Geometry check sheet. Reference: the model listing, model coordinates, mm. A direction names the side the tool comes from. Round coordinates to 2 decimals unless told otherwise and drop trailing zeros. Loops run counter-clockwise (first coordinate to the right, second up) from the corner with the lowest first, then second, coordinate; pieces in that order, holes last.
```python
from build123d import *

# Parameters (mm, degrees)
F0_R     = 15.875
F1_DEPTH = 31.75
F2_DEPTH = 92.075
F0_W     = 31.75
F0_H     = 88.9
F3_DEPTH = 73.025
F4_DEPTH = 53.975


# Not quite as in the source:
# - a feature names something its author has since deleted; it is built from what else it names


with BuildPart() as f1:
    # F0 (on Front) → F1 (new body)
    with BuildSketch(Plane.XZ):
        Polygon((-69.8361151936, 86.826035718), (-126.218325014, 80.5985571647), (-126.4791783958, 29.7122203269), (-85.725, 29.7122203269), (-85.725, -21.0877796731), (-126.7395891979, -21.0877796731), (-127, -71.8877796731), (-69.8361151936, -65.5739758634), (-69.8361151936, -40.1377796731), (-69.8361151936, 48.7622203269), align=None)
        Polygon((126.2463778257, 108.4835678339), (-69.8361151936, 86.826035718), (-69.8361151936, 48.7622203269), (-38.0861151936, 48.7622203269), (-38.0861151936, -40.1377796731), (-38.0861151936, -62.0671590745), (38.1138848064, -53.6507987812), (38.1138848064, -40.1378311361), (38.1138848064, 48.7622203269), (69.8638848064, 48.7622203269), (69.8638848064, -40.1378311361), (69.8638848064, -50.1439819923), (126.2463778257, -43.9164836263), (126.2463778257, 6.8835678339), (85.725, 6.8835678339), (85.725, 57.6835678339), (126.2463778257, 57.6835678339), align=None)
        Circle(F0_R, mode=Mode.SUBTRACT)
        Polygon((-38.0861151936, -40.1377796731), (-69.8361151936, -40.1377796731), (-69.8361151936, -65.5739758634), (-38.0861151936, -62.0671590745), align=None)
    extrude(amount=F1_DEPTH)

    # F0 (on Front) → F2 (join)
    with BuildSketch(Plane.XZ):
        Polygon((126.2463778257, 108.4835678339), (-69.8361151936, 86.826035718), (-69.8361151936, 48.7622203269), (-38.0861151936, 48.7622203269), (-38.0861151936, -40.1377796731), (-38.0861151936, -62.0671590745), (38.1138848064, -53.6507987812), (38.1138848064, -40.1378311361), (38.1138848064, 48.7622203269), (69.8638848064, 48.7622203269), (69.8638848064, -40.1378311361), (69.8638848064, -50.1439819923), (126.2463778257, -43.9164836263), (126.2463778257, 6.8835678339), (85.725, 6.8835678339), (85.725, 57.6835678339), (126.2463778257, 57.6835678339), align=None)
        Circle(F0_R, mode=Mode.SUBTRACT)
        Polygon((-38.0861151936, -40.1377796731), (-69.8361151936, -40.1377796731), (-69.8361151936, -65.5739758634), (-38.0861151936, -62.0671590745), align=None)
        Polygon((38.1138848064, -40.1378311361), (38.1138848064, -53.6507987812), (69.8638848064, -50.1439819923), (69.8638848064, -40.1378311361), align=None)
    extrude(amount=F2_DEPTH)

    # F0 (on Front) → F3 (join)
    with BuildSketch(Plane.XZ):
        with Locations((-53.9611151936, 4.3122203269)):
            Rectangle(F0_W, F0_H)
    extrude(amount=F3_DEPTH)

    # F0 (on Front) → F4 (join)
    with BuildSketch(Plane.XZ):
        Polygon((126.2463778257, 108.4835678339), (-69.8361151936, 86.826035718), (-69.8361151936, 48.7622203269), (-38.0861151936, 48.7622203269), (-38.0861151936, -40.1377796731), (-38.0861151936, -62.0671590745), (38.1138848064, -53.6507987812), (38.1138848064, -40.1378311361), (38.1138848064, 48.7622203269), (69.8638848064, 48.7622203269), (69.8638848064, -40.1378311361), (69.8638848064, -50.1439819923), (126.2463778257, -43.9164836263), (126.2463778257, 6.8835678339), (85.725, 6.8835678339), (85.725, 57.6835678339), (126.2463778257, 57.6835678339), align=None)
        Circle(F0_R, mode=Mode.SUBTRACT)
    extrude(amount=F4_DEPTH)


solid = f1.part
```
1) Gauge pin test, flat ends, axial feed: pin 1 (21 mm diameter, centred on x = -49.5, y = -78, fed in from -Z); pin 2 (5 mm diameter, centred on x = 47.5, y = -26.5, fed in from -Z); pin 3 (16 mm diameter, centred on x = -110.5, y = -9.5, fed in from -Z). Record the tip position at first contact, or that the pin passes through.
Report:
pin 1: stops at z = -64.49
pin 2: stops at z = -52.89
pin 3: stops at z = -70.95
2) Scan lines: line 1 along X through (y, z) = (-38.5, -29); line 2 along X through (y, z) = (-46.5, -5); line 3 along X through (y, z) = (-38, -7.5). Record each from-to range of solid material in increasing order.
Report:
line 1: x = -69.84 to 38.11, 69.86 to 126.25
line 2: x = -69.84 to -15.07, 15.07 to 38.11, 69.86 to 126.25
line 3: x = -69.84 to -13.99, 13.99 to 38.11, 69.86 to 126.25
3) Mould release check, pull along Z, two halves, no side actions. Record for faces 6 (the face through (126.246, -45, -19)), 7 (the face through (-38.086, -82, 5)), 8 (the face through (25.99, -45.39, -54.99)), 9 (the face through (-85.725, -16, 5)): +Z half, -Z half, draft (parallel to the pull), parting line (faces both ways), or undercut.
Report:
face 6: draft
face 7: undercut
face 8: -Z half
face 9: undercut
4) Access from +Z, -Z, +X, -X, +Y, -Y to the whole of each face (thin tool, end or side, straight path). Record for faces 1 (the face through (-69.836, -55, 10)), 2 (the face through (54, -45, -40.138)), 3 (the face through (-54, -82, 48.762)), 4 (the face through (106, -45, 57.684)), 5 (the face through (-106, -16, -21.088)).
Report:
face 1: +Z, -Z, -X, -Y
face 2: +Y, -Y
face 3: -X, -Y
face 4: +X, +Y, -Y
face 5: -X, +Y, -Y
5) Sectioned sample at A-A, the plane y = -57.5. Record the cut outline in (x, z) (3 decimals).
Report:
outline: (-69.836, -65.574) - (126.246, -43.916) - (126.246, 6.884) - (85.725, 6.884) - (85.725, 57.684) - (126.246, 57.684) - (126.246, 108.484) - (-69.836, 86.826) - close; hole circle Ø31.75 at (0, 0); hole (38.114, -40.138) - (69.864, -40.138) - (69.864, 48.762) - (38.114, 48.762) - close
6) Sectioned sample at D-D, the plane z = 34. Record the cut outline in (x, y) (3 decimals), then the cut area to 3 significant figures.
Report:
outline: (-126.457, -31.75) - (-69.836, -31.75) - (-69.836, -73.025) - (-38.086, -73.025) - (-38.086, -92.075) - (38.114, -92.075) - (38.114, 0) - (-126.457, 0) - close; (69.864, -92.075) - (85.725, -92.075) - (85.725, 0) - (69.864, 0) - close
area: 12,600 mm2
7) Sectioned sample at B-B, the plane z = 0. Record the cut outline in (x, y) (3 decimals).
Report:
outline: (-85.725, -31.75) - (-69.836, -31.75) - (-69.836, -73.025) - (-38.086, -73.025) - (-38.086, -92.075) - (-15.875, -92.075) - (-15.875, 0) - (-85.725, 0) - close; (15.875, -92.075) - (38.114, -92.075) - (38.114, 0) - (15.875, 0) - close; (69.864, -92.075) - (126.246, -92.075) - (126.246, 0) - (69.864, 0) - close
8) Sectioned sample at C-C, the plane x = 13. Record the cut outline in (y, z) (3 decimals).
Report:
outline: (-92.075, -56.425) - (0, -56.425) - (0, -9.111) - (-92.075, -9.111) - close; (-92.075, 9.111) - (0, 9.111) - (0, 95.975) - (-92.075, 95.975) - close
